from build123d import *

# Parameters (mm, degrees)
SKETCH4_W                      = 116
SKETCH4_H                      = 116
BOSS_EXTRUDE1_DEPTH            = 4
SKETCH6_R                      = 30
CUT_EXTRUDE1_DEPTH             = 83.121860671
BOSS_EXTRUDE3_DEPTH            = 8.4
SKETCH10_W                     = 116
SKETCH10_H                     = 116
BOSS_EXTRUDE5_DEPTH            = 15
SKETCH11_R                     = 4
POSITIONING_HOLE_DEPTH         = 26
SKETCH23_R                     = 4
SNAPPING_HOLE_DEPTH            = 26
SKETCH13_R                     = 31.25
SKETCH13_R_2                   = 30
BOSS_EXTRUDE6_DEPTH            = 25
SKETCH24_W                     = 40
SKETCH24_H                     = 8
BOSS_EXTRUDE7_DEPTH            = 150
BOSS_EXTRUDE9_DEPTH            = 40
CUT_EXTRUDE6_DEPTH             = 8
CUT_EXTRUDE6_DIRECTION_2_REACH = 229.876
CUT_EXTRUDE7_REACH             = 225.194
CUT_EXTRUDE9_REACH             = 204.284
SKETCH37_W                     = 25
SKETCH37_H                     = 20
SKETCH41_W                     = 210
SKETCH41_H                     = 210
BOSS_EXTRUDE11_DEPTH           = 5
SKETCH12_R                     = 30
MAIN_HOLE_DEPTH                = 212.068709192
SKETCH43_W                     = 8
SKETCH43_H                     = 8
SKETCH43_R                     = 2
BOSS_EXTRUDE12_DEPTH           = 5


with BuildPart() as part:
    # Sketch4 → Boss-Extrude1 (new body)
    with BuildSketch(Plane(origin=(0, 0, 0), x_dir=(1, 0, 0), z_dir=(0, 1, 0))):
        Rectangle(SKETCH4_W, SKETCH4_H)
    extrude(amount=BOSS_EXTRUDE1_DEPTH)

    # Sketch6 → Cut-Extrude1 (cut, through all)
    with BuildSketch(Plane(origin=(0, 4, 0), x_dir=(1, 0, 0), z_dir=(0, 1, 0))):
        with Locations(Location((0, 0, 0), (0, 0, 270))):
            Circle(SKETCH6_R)
    extrude(amount=-CUT_EXTRUDE1_DEPTH, mode=Mode.SUBTRACT)

    # Sketch8 → Boss-Extrude3 (add)
    with BuildSketch(Plane.XZ):
        with BuildLine():
            Line((-58, 58), (-58, -58))
            Line((-58, -58), (22, -58))
            ThreePointArc((22, -58), (-36, 0), (22, 58))
            Line((22, 58), (-58, 58))
        make_face()
    extrude(amount=BOSS_EXTRUDE3_DEPTH)

    # Sketch10 → Boss-Extrude5 (add)
    with BuildSketch(Plane.XZ.offset(8.4)):
        Rectangle(SKETCH10_W, SKETCH10_H)
    extrude(amount=BOSS_EXTRUDE5_DEPTH)

    # Sketch11 → positioning hole (cut)
    with BuildSketch(Plane.XZ.offset(23.4)):
        with Locations(Location((39, 0, 0), (0, 0, 270))):
            Circle(SKETCH11_R)
    extrude(amount=-POSITIONING_HOLE_DEPTH, mode=Mode.SUBTRACT)

    # Sketch23 → snapping hole (cut)
    with BuildSketch(Plane.XZ.offset(23.4)):
        with Locations(Location((38.947036647, 20, 0), (0, 0, 270))):
            Circle(SKETCH23_R)
    extrude(amount=-SNAPPING_HOLE_DEPTH, mode=Mode.SUBTRACT)

    # Sketch13 → Boss-Extrude6 (add)
    with BuildSketch(Plane.XZ.offset(23.4)):
        with Locations(Location((0, 0, 0), (0, 0, 270))):
            Circle(SKETCH13_R)
        with Locations(Location((0, 0, 0), (0, 0, 90))):
            Circle(SKETCH13_R_2, mode=Mode.SUBTRACT)
    extrude(amount=BOSS_EXTRUDE6_DEPTH)

    # Sketch24 → Boss-Extrude7 (add)
    with BuildSketch(Plane.XZ.offset(23.4)):
        with Locations((0, 54)):
            Rectangle(SKETCH24_W, SKETCH24_H)
        with Locations((0, -54)):
            Rectangle(SKETCH24_W, SKETCH24_H)
    extrude(amount=BOSS_EXTRUDE7_DEPTH)

    # Sketch28 → Boss-Extrude9 (add)
    with BuildSketch(Plane.ZY.offset(20)):
        Polygon((-58, -173.4), (-58, 4), (-78, 4), align=None)
        Polygon((58, 4), (58, -173.4), (78, 4), align=None)
    extrude(amount=-BOSS_EXTRUDE9_DEPTH)

    # Sketch31 → Cut-Extrude6 (cut)
    with BuildSketch(Plane(origin=(0, 0, -58), x_dir=(-1, 0, 0), z_dir=(0, 0, -1))):
        with BuildLine():
            Line((2.5, -28.4), (2.5, -168.4))
            ThreePointArc((2.5, -168.4), (0, -170.9), (-2.5, -168.4))
            Line((-2.5, -168.4), (-2.5, -28.4))
            ThreePointArc((-2.5, -28.4), (0, -25.9), (2.5, -28.4))
        make_face()
    extrude(amount=-CUT_EXTRUDE6_DEPTH, mode=Mode.SUBTRACT)

    # Cut-Extrude6 direction 2: up to this plane
    cut_extrude6_direction_2_end = Plane(origin=(20, 4, -78), z_dir=(0, -0.11202985805393491, -0.9937048409384023))
    # Sketch31 → Cut-Extrude6 direction 2 (cut, up to the surface)
    with BuildSketch(Plane(origin=(0, 0, -58), x_dir=(-1, 0, 0), z_dir=(0, 0, -1)), mode=Mode.PRIVATE) as cut_extrude6_direction_2_sk1:
        with BuildLine():
            Line((2.5, -28.4), (2.5, -168.4))
            ThreePointArc((2.5, -168.4), (0, -170.9), (-2.5, -168.4))
            Line((-2.5, -168.4), (-2.5, -28.4))
            ThreePointArc((-2.5, -28.4), (0, -25.9), (2.5, -28.4))
        make_face()
    cut_extrude6_direction_2_tool1 = split(extrude(cut_extrude6_direction_2_sk1.sketch, amount=CUT_EXTRUDE6_DIRECTION_2_REACH, mode=Mode.PRIVATE), bisect_by=cut_extrude6_direction_2_end, keep=Keep.BOTH, mode=Mode.PRIVATE)
    add(cut_extrude6_direction_2_tool1.solids().sort_by_distance((0, -98.4, -58))[0], mode=Mode.SUBTRACT)

    # Cut-Extrude7: up to this plane
    cut_extrude7_end = Plane(origin=(20, -173.4, 58), z_dir=(0, -0.11202985805393491, 0.9937048409384023))
    # Sketch34 → Cut-Extrude7 (cut, up to the surface)
    with BuildSketch(Plane(origin=(0, 0, 50), x_dir=(-1, 0, 0), z_dir=(0, 0, -1)), mode=Mode.PRIVATE) as cut_extrude7_sk1:
        with BuildLine():
            Line((-2.5, -28.4), (-2.5, -168.4))
            ThreePointArc((-2.5, -168.4), (0, -170.9), (2.5, -168.4))
            Line((2.5, -168.4), (2.5, -28.4))
            ThreePointArc((2.5, -28.4), (0, -25.9), (-2.5, -28.4))
        make_face()
    cut_extrude7_tool1 = split(extrude(cut_extrude7_sk1.sketch, amount=-CUT_EXTRUDE7_REACH, mode=Mode.PRIVATE), bisect_by=cut_extrude7_end, keep=Keep.BOTH, mode=Mode.PRIVATE)
    add(cut_extrude7_tool1.solids().sort_by_distance((0, -98.4, 50))[0], mode=Mode.SUBTRACT)

    # Sketch37 → Cut-Extrude9 (cut, up to next)
    with BuildSketch(Plane(origin=(0, 4, 0), x_dir=(1, 0, 0), z_dir=(0, 1, 0)), mode=Mode.PRIVATE) as cut_extrude9_sk1:
        with Locations((0, 68)):
            Rectangle(SKETCH37_W, SKETCH37_H)
    cut_extrude9_tool1 = extrude(cut_extrude9_sk1.sketch, amount=-CUT_EXTRUDE9_REACH, mode=Mode.PRIVATE) & part.part
    # Sketch37 → Cut-Extrude9 (cut, up to next)
    with BuildSketch(Plane(origin=(0, 4, 0), x_dir=(1, 0, 0), z_dir=(0, 1, 0)), mode=Mode.PRIVATE) as cut_extrude9_sk2:
        with Locations((0, -68)):
            Rectangle(SKETCH37_W, SKETCH37_H)
    cut_extrude9_tool2 = extrude(cut_extrude9_sk2.sketch, amount=-CUT_EXTRUDE9_REACH, mode=Mode.PRIVATE) & part.part
    add(cut_extrude9_tool1.solids().sort_by_distance((0, 4, -68))[0], mode=Mode.SUBTRACT)
    add(cut_extrude9_tool2.solids().sort_by_distance((0, 4, 68))[0], mode=Mode.SUBTRACT)

    # Sketch41 → Boss-Extrude11 (add)
    with BuildSketch(Plane(origin=(0, 4, 0), x_dir=(1, 0, 0), z_dir=(0, 1, 0))):
        Rectangle(SKETCH41_W, SKETCH41_H)
    extrude(amount=BOSS_EXTRUDE11_DEPTH)

    # Sketch12 → main hole (cut, through all)
    with BuildSketch(Plane.XZ.offset(23.4)):
        with Locations(Location((0, 0, 0), (0, 0, 90))):
            Circle(SKETCH12_R)
    extrude(amount=-MAIN_HOLE_DEPTH, mode=Mode.SUBTRACT)

    # Sketch43 → Boss-Extrude12 (add)
    # profile 1 of 4: a face of its own
    with BuildSketch(Plane(origin=(0, 9, 0), x_dir=(1, 0, 0), z_dir=(0, 1, 0))):
        with Locations((101, 109)):
            Rectangle(SKETCH43_W, SKETCH43_H)
        with Locations(Location((101, 109, 0), (0, 0, 270))):
            Circle(SKETCH43_R, mode=Mode.SUBTRACT)
    # profile 2 of 4: a face of its own
    with BuildSketch(Plane(origin=(0, 9, 0), x_dir=(1, 0, 0), z_dir=(0, 1, 0))):
        with Locations((-101, 109)):
            Rectangle(SKETCH43_W, SKETCH43_H)
        with Locations(Location((-101, 109, 0), (0, 0, 270))):
            Circle(SKETCH43_R, mode=Mode.SUBTRACT)
    # profile 3 of 4: a face of its own
    with BuildSketch(Plane(origin=(0, 9, 0), x_dir=(1, 0, 0), z_dir=(0, 1, 0))):
        with Locations((-101, -109)):
            Rectangle(SKETCH43_W, SKETCH43_H)
        with Locations(Location((-101, -109, 0), (0, 0, 90))):
            Circle(SKETCH43_R, mode=Mode.SUBTRACT)
    # profile 4 of 4: a face of its own
    with BuildSketch(Plane(origin=(0, 9, 0), x_dir=(1, 0, 0), z_dir=(0, 1, 0))):
        with Locations((101, -109)):
            Rectangle(SKETCH43_W, SKETCH43_H)
        with Locations(Location((101, -109, 0), (0, 0, 90))):
            Circle(SKETCH43_R, mode=Mode.SUBTRACT)
    extrude(amount=-BOSS_EXTRUDE12_DEPTH)


solid = part.part
Input: part model. Units: mm. Frame: model coordinates. A direction names the side the tool comes from. Give positions to 0.01 mm unless a question says otherwise; leave off trailing zeros. Order: outer loops, then holes, each group sorted by start corner. A loop starts at its lowest first (then second) coordinate and runs counter-clockwise, first axis right, second up. Notation, with made-up numbers: (71.25, -11) - (124.25, -11) arc R31 ccw to (124.25, 26) - close; hole circle Ø5 at (61.5, 1). An arc over 180 degrees is marked (long way). Answer as a JSON object with one key per item and string values. Group by question number.
Q1. Cut plane D-D, the plane x = -63. Output: boundary loops of the cut face in (y, z), then the cut area to 3 significant figures.
Q2. Cut plane A-A, the plane z = 0. Count the separate pieces of the cut face and the enclosed holes in it, then the cut area to 3 significant figures.
Q3. First-contact query: pin 1 Ø12.5 at (x, y) = (-5.5, -89.5) entering from -Z; pin 2 Ø2.5 at (x, y) = (-19, 7.5) entering from +Z; pin 3 Ø4 at (x, z) = (65.5, -45.5) entering from -Y. Flat tips, straight axial feed; report the tip coordinate or a pass-through.
Q4. Line query: probe 1 along X at (y, z) = (5.75, -109); probe 2 along X at (y, z) = (1, 0); probe 3 along X at (y, z) = (-103.5, 52.5). Output: solid intervals per line, ascending.
Q5. Cut plane B-B, the plane y = -153. Output: boundary loops of the cut face in (x, z).
Q6. Cut plane C-C, the plane z = -93.5. Output: boundary loops of the cut face in (x, y).
Q7. Set-up query: faces 1 (the face through (58, -16, -1)), 2 (the face through (39, -13, -58)), 3 (the face through (-35.986, -4.141, -1.275)), 4 (the face through (-12.5, -44, 64)). Return all of +Z, -Z, +X, -X, +Y, -Y with unobstructed straight access to the full face (end or side cutting, diameter ignored); none if empty.
Q8. Mould query, pull axis Z, two halves, no side actions, for faces 5 (the face through (39, 2.6, 20)), 6 (the face through (-71, 4, -2)), 7 (the face through (-39, -10, -58)). Classes: pulls with the +Z half, pulls with the -Z half, needs draft (parallel to the pull), parting line crosses it, or undercut.
Results:
{
 "1": {"outline": "(4, -105) - (9, -105) - (9, 105) - (4, 105) - close", "area": "1,050 mm^2"},
 "2": {"separate pieces": "4", "enclosed holes": "0", "area": "1,920 mm^2"},
 "3": {"pin 1": "z = -58", "pin 2": "z = 105", "pin 3": "y = 4"},
 "4": {"probe 1": "-105 to -103, -99 to -97, 97 to 99, 103 to 105", "probe 2": "-58 to -30, 30 to 35, 43 to 58", "probe 3": "-20 to -2.5, 2.5 to 20"},
 "5": {"outline": "(-20, -60.3) - (-12.5, -60.3) - (-12.5, -58) - (-2.5, -58) - (-2.5, -50) - (-20, -50) - close; (-20, 50) - (-2.5, 50) - (-2.5, 58) - (-12.5, 58) - (-12.5, 60.3) - (-20, 60.3) - close; (2.5, -58) - (12.5, -58) - (12.5, -60.3) - (20, -60.3) - (20, -50) - (2.5, -50) - close; (2.5, 50) - (20, 50) - (20, 60.3) - (12.5, 60.3) - (12.5, 58) - (2.5, 58) - close"},
 "6": {"outline": "(-105, 4) - (105, 4) - (105, 9) - (-105, 9) - close"},
 "7": {"face 1": "+Z, -Z, +X, -Y", "face 2": "-Z, +X, -Y", "face 3": "+X", "face 4": "+Z, -Y"},
 "8": {"face 5": "undercut", "face 6": "needs draft", "face 7": "pulls with the -Z half"}
}
